For this review, take the finished solid that the model builds, in its own axes (mm). Give positions to 0.01 mm unless a question says otherwise; leave off trailing zeros. Loops run counter-clockwise (first coordinate to the right, second up) from the corner with the lowest first, then second, coordinate; pieces in that order, holes last.
```python
from build123d import *

# Parameters (mm, degrees)
SZKIC1_R                    = 6
SZKIC1_R_2                  = 4.5
DODANIE_WYCI_GNI_CIE1_DEPTH = 6


with BuildPart() as part:
    # Szkic1 → Dodanie-wyciągnięcie1 (new body)
    with BuildSketch(Plane.XY):
        with BuildLine():
            Line((-47, 152.941165158), (-47, -152.941165158))
            ThreePointArc((-47, -152.941165158), (0, -160), (47, -152.941165158))
            Line((47, -152.941165158), (47, 152.941165158))
            ThreePointArc((47, 152.941165158), (0, 160), (-47, 152.941165158))
        make_face()
        Circle(SZKIC1_R, mode=Mode.SUBTRACT)
        with Locations((0, -70)):
            Circle(SZKIC1_R_2, mode=Mode.SUBTRACT)
        with Locations((0, 70)):
            Circle(SZKIC1_R_2, mode=Mode.SUBTRACT)
        with Locations((0, 135)):
            Circle(SZKIC1_R_2, mode=Mode.SUBTRACT)
        with Locations((0, -135)):
            Circle(SZKIC1_R_2, mode=Mode.SUBTRACT)
    extrude(amount=DODANIE_WYCI_GNI_CIE1_DEPTH)


solid = part.part
```
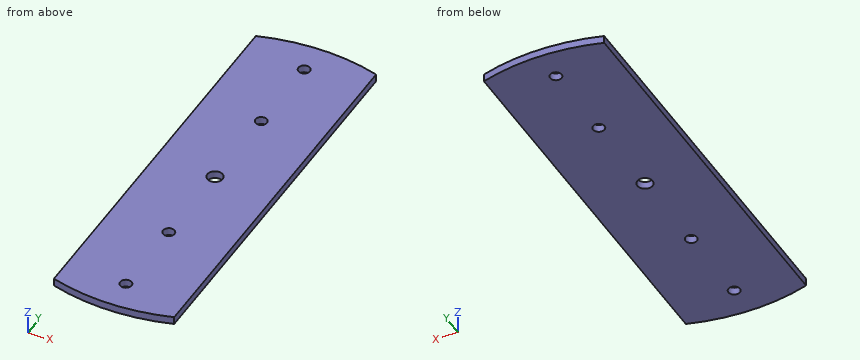
Item 1: Take a section at D-D on y = 135. Give the boundary of the cut face in (x, z), and give its area (3 significant figures).
Answer:
outline: (-47, 0) - (-4.5, 0) - (-4.5, 6) - (-47, 6) - close; (4.5, 0) - (47, 0) - (47, 6) - (4.5, 6) - close
area: 510 mm2
Item 2: Take a section at B-B on x = 0. Give the boundary of the cut face in (y, z).
Answer:
outline: (-160, 0) - (-139.5, 0) - (-139.5, 6) - (-160, 6) - close; (-130.5, 0) - (-74.5, 0) - (-74.5, 6) - (-130.5, 6) - close; (-65.5, 0) - (-6, 0) - (-6, 6) - (-65.5, 6) - close; (6, 0) - (65.5, 0) - (65.5, 6) - (6, 6) - close; (74.5, 0) - (130.5, 0) - (130.5, 6) - (74.5, 6) - close; (139.5, 0) - (160, 0) - (160, 6) - (139.5, 6) - close
Item 3: For L1, parallel to X at y = 3, z = 5.1; L2, parallel to X at y = 71, z = 5.3; L3, parallel to Y at x = 43, z = 3.7, list the stretches that pass through material, from the lowest coordinate up.
Answer:
L1: x = -47 to -5.2, 5.2 to 47
L2: x = -47 to -4.39, 4.39 to 47
L3: y = -154.11 to 154.11
Item 4: Clearance check with flat-ended pins moving along their axes: pin 1 Ø1.5 at (x, z) = (17.5, 3.5) entering from -Y; pin 2 Ø1.5 at (x, z) = (27, 3.5) entering from +Y. State where each tip first meets the part, or that it passes through.
Answer:
pin 1: stops at y = -159.12
pin 2: stops at y = 157.83
Item 5: Take a section at C-C on z = 4.75. Give the boundary of the cut face in (x, y).
Answer:
outline: (-47, -152.94) arc R160 ccw to (47, -152.94) - (47, 152.94) arc R160 ccw to (-47, 152.94) - close; hole circle Ø12 at (0, 0); hole circle Ø9 at (0, -135); hole circle Ø9 at (0, -70); hole circle Ø9 at (0, 70); hole circle Ø9 at (0, 135)
Item 6: Take a section at A-A on y = 0. Give the boundary of the cut face in (x, z), and give its area (3 significant figures).
Answer:
outline: (-47, 0) - (-6, 0) - (-6, 6) - (-47, 6) - close; (6, 0) - (47, 0) - (47, 6) - (6, 6) - close
area: 492 mm2
